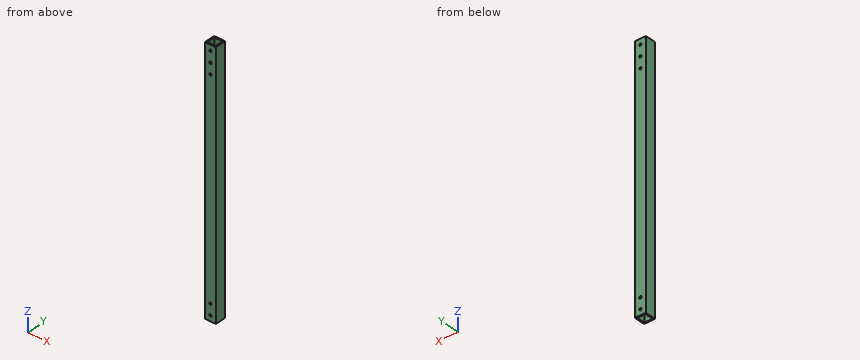
Autodesk Inventor part; units mm, degrees
ref_plane "YZ Plane" through (0, 0, 0) normal (1, 0, 0) x (0, 1, 0)
ref_plane "XZ Plane" through (0, 0, 0) normal (0, 1, 0) x (-1, 0, 0)
ref_plane "XY Plane" through (0, 0, 0) normal (0, 0, 1) x (1, 0, 0)
sketch "Sketch1" plane through (0, 0, 0) normal (0, 0, 1) x (1, 0, 0)
  line L0 (0, 0) -> (25.4, 0)
  line L1 (25.4, 0) -> (25.4, 25.4)
  line L2 (25.4, 25.4) -> (0, 25.4)
  line L3 (0, 25.4) -> (0, 0)
  line L4 (3.175, 22.225) -> (22.225, 22.225)
  line L5 (22.225, 22.225) -> (22.225, 3.175)
  line L6 (22.225, 3.175) -> (3.175, 3.175)
  line L7 (3.175, 3.175) -> (3.175, 22.225)
  dimension "d0" = 25.4
  dimension "d1" = 25.4
  dimension "d2" = 3.175
extrude "Extrusion1" add sketch "Sketch1" against normal blind 590.55
sketch "Sketch5" plane through (0, 25.4, 0) normal (0, 1, 0) x (1, 0, 0)
  line L0 (25.4, 590.55) -> (0, 590.55)
  line L1 (25.4, 0) -> (0, 0)
  point P0 (12.7, 12.7)
  point P1 (12.7, 38.1)
  point P2 (12.7, 63.5)
  point P3 (12.7, 577.85)
  point P4 (12.7, 552.45)
  dimension "d32" = 12.7
  dimension "d33" = 25.4
  dimension "d34" = 12.7
  dimension "d35" = 25.4
  dimension "d36" = 25.4
hole "Hole4" at (12.7, 25.4, -12.7) at (12.7, 25.4, -38.1) at (12.7, 25.4, -63.5) at (12.7, 25.4, -577.85) at (12.7, 25.4, -552.45) direction (0, -1, 0) diameter 5.334 depth 25.4 tip angle 118
properties part number "new horizontal kicker thingleft"
Design review of the part built by this model. Coordinates are the model's own, in mm. Coordinates: 2 decimals unless noted, no trailing zeros. Order: outer loops, then holes, each group sorted by start corner. A loop starts at its lowest first (then second) coordinate and runs counter-clockwise, first axis right, second up.
Item 1: Take a section at B-B, the plane z = -518. Write out the cut boundary in (x, y) (3 decimals).
Item 2: For line 1 (Z direction, x = 12.7, y = 23.55); line 2 (Y direction, x = 19.25, z = -488.5) (3 decimals); line 3 (X direction, y = 23.35, z = -552.45), list the stretches that pass through material, from the lowest coordinate up.
Item 3: Take a section at A-A, the plane y = 14. Write out the cut boundary in (x, z) (3 decimals).
The answers:
1. outline: (0, 0) - (25.4, 0) - (25.4, 25.4) - (0, 25.4) - close; hole (3.175, 3.175) - (22.225, 3.175) - (22.225, 22.225) - (3.175, 22.225) - close
2. line 1: z = -590.55 to -580.52, -575.18 to -555.12, -549.78 to -66.17, -60.83 to -40.77, -35.43 to -15.37, -10.03 to 0
2. line 2: y = 0 to 3.175, 22.225 to 25.4
2. line 3: x = 0 to 10.03, 15.37 to 25.4
3. outline: (0, -590.55) - (3.175, -590.55) - (3.175, 0) - (0, 0) - close; (22.225, -590.55) - (25.4, -590.55) - (25.4, 0) - (22.225, 0) - close
